Part model, mm, in its own coordinate system. A direction names the side the tool comes from. Coordinates: 2 decimals unless noted, no trailing zeros. Loops run counter-clockwise (first coordinate to the right, second up) from the corner with the lowest first, then second, coordinate; pieces in that order, holes last. Notation, with made-up numbers: M 50,87 L 70,87 A15 ccw 70,109 Z; hole C 71.5,31.25 d3. An arc over 180 degrees is marked long. Use a Markdown table: item, result. Add a question column.
1) Band-saw the part on A-A (x = 0). List the corners of the cut face in (y, z), plus the area to 3 significant figures.
2) Band-saw the part on D-D (x = 24). List the corners of the cut face in (y, z), plus the area to 3 significant figures.
3) Wall check: probe 1 along Y at (x, z) = (0, -29); probe 2 along Y at (x, z) = (22, 3); probe 3 along Z at (x, y) = (24, 38). Give the ranges that are in metal, low to high. Write a range as from..to.
4) Band-saw the part on C-C (z = 4.5). List the corners of the cut face in (x, y).
5) Tool access for faces 4 (the flat face through (34.5, 47.73, -29.25)), 5 (the flat face through (-1, 9.1, 6)): list every direction of +Z, -Z, +X, -X, +Y, -Y with a clear straight run to the whole face (end or side of a thin tool).
6) Pull direction Y, two halves, no side cores. Call faces 1 (the flat face through (-34.06, 48.82, -29.25)), 2 (the cylindrical face through (-1.15, 77.78, -29.05)), 3 (the flat face through (-1, 4, 32.5)): released by +Y, released by -Y, zero draft, split by the parting line, or undercut.
7) Pin check, flat tips, straight feed: pin 1 Ø4 at (x, z) = (11, 7) entering from +Y; pin 2 Ø4.5 at (x, y) = (0, 43) entering from -Z; pin 3 Ø3 at (x, y) = (9, 46) entering from +Z. Stop position of each tip, or through.
8) Band-saw the part on B-B (y = 80). List the corners of the cut face in (x, z), plus the area to 3 significant figures.
from build123d import *

# Parameters (mm, degrees)
SKETCH1_W                 = 100
SKETCH1_H                 = 65
EXTRUDE1_DEPTH            = 9.1
EXTRUDE2_DEPTH            = 7
M6X1_0_TAPPED_HOLE2_D     = 5
M6X1_0_TAPPED_HOLE2_DEPTH = 15
M6X1_0_TAPPED_HOLE2_TIP   = 1.502151548
FILLET1_R                 = 5
FILLET2_R                 = 5


with BuildPart() as part:
    # Sketch1 → Extrude1 (new body)
    with BuildSketch(Plane(origin=(0, 0, 0), x_dir=(1, 0, 0), z_dir=(0, 1, 0))):
        Rectangle(SKETCH1_W, SKETCH1_H)
    extrude(amount=EXTRUDE1_DEPTH)

    # Sketch3 → Extrude2 (add)
    with BuildSketch(Plane(origin=(0, 0, -32.5), x_dir=(-1, 0, 0), z_dir=(0, 0, -1))):
        with BuildLine():
            Line((-50, 9.1), (-18.561406243, 87.448100313))
            ThreePointArc((-18.561406243, 87.448100313), (0, 100), (18.561406243, 87.448100313))
            Line((18.561406243, 87.448100313), (50, 9.1))
            Line((50, 9.1), (-50, 9.1))
        make_face()
    extrude(amount=-EXTRUDE2_DEPTH)

    # M6x1.0 Tapped Hole2
    with Locations(Plane.XY.offset(-25.5)):
        with Locations((0, 80), (0, 43)):
            Hole(M6X1_0_TAPPED_HOLE2_D / 2, depth=M6X1_0_TAPPED_HOLE2_DEPTH)
            with Locations((0, 0, -(M6X1_0_TAPPED_HOLE2_DEPTH + M6X1_0_TAPPED_HOLE2_TIP / 2))):  # 118° drill point
                Cone(0, M6X1_0_TAPPED_HOLE2_D / 2, M6X1_0_TAPPED_HOLE2_TIP, mode=Mode.SUBTRACT)

    # Fillet1
    fillet1_edges = [part.edges().sort_by_distance(p)[0] for p in [
        (0, 9.1, -25.5),
    ]]
    fillet(fillet1_edges, radius=FILLET1_R)

    # Fillet2
    fillet2_edges = [part.edges().sort_by_distance(p)[0] for p in [
        (-50, 4.55, 32.5),
        (50, 4.55, 32.5),
    ]]
    fillet(fillet2_edges, radius=FILLET2_R)


solid = part.part
Entries:
| question | item | result |
|---|---|---|
| 1 | outline | M 0,-32.5 L 40.5,-32.5 L 40.5,-25.5 L 14.1,-25.5 A5 cw 9.1,-20.5 L 9.1,32.5 L 0,32.5 Z; M 45.5,-32.5 L 77.5,-32.5 L 77.5,-25.5 L 45.5,-25.5 Z; M 82.5,-32.5 L 100,-32.5 L 100,-25.5 L 82.5,-25.5 Z |
| 1 | area | 1,160 mm2 |
| 2 | outline | M 0,-32.5 L 73.89,-32.5 L 73.89,-25.5 L 14.1,-25.5 A5 cw 9.1,-20.5 L 9.1,32.5 L 0,32.5 Z |
| 2 | area | 1,050 mm2 |
| 3 | probe 1 | 0..40.5, 45.5..77.5, 82.5..100 |
| 3 | probe 2 | 0..9.1 |
| 3 | probe 3 | -32.5..-25.5 |
| 4 | outline | M -50,0 L 50,0 L 50,9.1 L -50,9.1 Z |
| 5 | face 4 | +Z, -Z, +X, +Y |
| 5 | face 5 | +Z, +X, -X, +Y |
| 6 | face 1 | released by +Y |
| 6 | face 2 | undercut |
| 6 | face 3 | zero draft |
| 7 | pin 1 | y = 9.1 |
| 7 | pin 2 | through |
| 7 | pin 3 | z = -25.5 |
| 8 | outline | M -21.55,-32.5 L -2.5,-32.5 L -2.5,-25.5 L -21.55,-25.5 Z; M 2.5,-32.5 L 21.55,-32.5 L 21.55,-25.5 L 2.5,-25.5 Z |
| 8 | area | 267 mm2 |
